The listing builds one solid part. Answer for the finished solid, in the listing's coordinates (mm). Round coordinates to 2 decimals unless told otherwise and drop trailing zeros. Write each loop counter-clockwise with the first axis right and the second up, starting at its lowest first coordinate (ties: lowest second). Pieces come first, ordered by that corner, then holes.
from build123d import *

# Parameters (mm, degrees)
F12_DEPTH = 3.175


with BuildPart() as f12:
    # F10 (on plane+point) → F12 (new body)
    with BuildSketch(Plane.XY.offset(179.6051224214)):
        with BuildLine():
            ThreePointArc((-1.5874999976, -0.9165435509), (-1.5875000012, -6.4158048657), (3.175, -3.6661742094))
            ThreePointArc((3.175, -3.6661742094), (2.7496306536, -2.0786742034), (1.5874999882, -0.9165435455))
            ThreePointArc((1.5874999882, -0.9165435455), (-5.4e-09, -0.4911742094), (-1.5874999976, -0.9165435509))
        make_face()
        with BuildLine():
            ThreePointArc((-1.5874999976, -0.9165435509), (-5.4e-09, -0.4911742094), (1.5874999882, -0.9165435455))
            ThreePointArc((1.5874999882, -0.9165435455), (0.4253693396, 0.2455871106), (0, 1.8330871047))
            ThreePointArc((0, 1.8330871047), (-0.4253693423, 0.2455871059), (-1.5874999976, -0.9165435509))
        make_face()
        with BuildLine():
            ThreePointArc((0, 1.8330871047), (0.4253693396, 0.2455871106), (1.5874999882, -0.9165435455))
            ThreePointArc((1.5874999882, -0.9165435455), (4.7624999941, -0.9165435558), (6.35, 1.8330871047))
            ThreePointArc((6.35, 1.8330871047), (3.175, 5.0080871047), (0, 1.8330871047))
        make_face()
        with BuildLine():
            ThreePointArc((0, 1.8330871047), (-5.9246306577, 3.4205871035), (-1.5874999976, -0.9165435509))
            ThreePointArc((-1.5874999976, -0.9165435509), (-0.4253693423, 0.2455871059), (0, 1.8330871047))
        make_face()
    extrude(amount=F12_DEPTH)


solid = f12.part
1. Straight lines are drawn through the part: line 1 along X through (y, z) = (-3.75, 182); line 2 along X through (y, z) = (4.25, 180.6); line 3 along X through (y, z) = (2.75, 181.55). For each, find the intervals that lie inside material, in ascending order.
Geometry says:
line 1: x = -3.17 to 3.17
line 2: x = -5.23 to -1.12, 1.12 to 5.23
line 3: x = -6.21 to -0.14, 0.14 to 6.21
2. For a pull along X with two mould halves and no side action, classify faces 1 (the face through (0, 0, 179.605)), 2 (the face through (-5.865, 3.52, 181.17)) as released by +X, released by -X, zero draft, split by the parting line, or undercut.
Geometry says:
face 1: zero draft
face 2: undercut
3. Section A-A on x = 2.5 is taken. Determine the outline of the cut face in (y, z).
Geometry says:
outline: (-5.62, 179.61) - (-1.71, 179.61) - (-1.71, 182.78) - (-5.62, 182.78) - close; (-1.27, 179.61) - (4.94, 179.61) - (4.94, 182.78) - (-1.27, 182.78) - close
4. Section B-B on y = 4 is taken. Determine the outline of the cut face in (x, z), plus the area to 3 significant figures.
Geometry says:
outline: (-5.5, 179.61) - (-0.85, 179.61) - (-0.85, 182.78) - (-5.5, 182.78) - close; (0.85, 179.61) - (5.5, 179.61) - (5.5, 182.78) - (0.85, 182.78) - close
area: 29.5 mm2
5. Section D-D on y = -4.5 is taken. Determine the outline of the cut face in (x, z).
Geometry says:
outline: (-3.06, 179.61) - (3.06, 179.61) - (3.06, 182.78) - (-3.06, 182.78) - close
6. Given pin 1 (1 mm diameter, centred on y = -4, z = 182, fed in from +X) (3 decimals); pin 2 (1 mm diameter, centred on y = -1, z = 181, fed in from -X), each flat-ended and moving along its own axis, determine where each tip first touches the part or whether it passes through.
Geometry says:
pin 1: stops at x = 3.175
pin 2: stops at x = -5.33
